Read the model definition and answer for the solid it produces. Units are mm, in the model's axes. A direction names the side the tool comes from. Coordinates: 2 decimals unless noted, no trailing zeros. Loops run counter-clockwise (first coordinate to the right, second up) from the corner with the lowest first, then second, coordinate; pieces in that order, holes last. Notation, with made-up numbers: (7.5, 36) - (44.5, 36) arc R29 cw to (44.5, 58) - close; hole circle Ø1 at (43, 53). An arc over 180 degrees is marked (long way). One line per item, written item: value. Start each with the question number.
from build123d import *

# Parameters (mm, degrees)
SKETCH_1_W               = 35
SKETCH_1_H               = 70
EXTRUDE_1_DEPTH          = 6
SKETCH_1_W_2             = 26
EXTRUDE_1_2_DEPTH        = 6
SKETCH_1_3_W             = 14
SKETCH_1_3_H             = 70
EXTRUDE_2_DEPTH          = 120
EXTRUDE_4_DEPTH          = 70
EXTRUDE_7_DEPTH          = 70
SKETCH_7_R               = 3
CUT_EXTRUDE_4_DEPTH      = 121
SKETCH_8_R               = 5
CUT_EXTRUDE_5_DEPTH      = 115
SKETCH_3_R               = 11.1
SKETCH_3_R_2             = 4.1
SKETCH_3_R_3             = 2
CUT_EXTRUDE_8_DEPTH      = 36
CUT_EXTRUDE_8_DEPTH_BACK = 41
SKETCH_10_W              = 75
SKETCH_10_H              = 24
EXTRUDE_8_DEPTH          = 6
SKETCH_11_R              = 3
CUT_EXTRUDE_9_DEPTH      = 6
SKETCH_12_W              = 56.46589335
SKETCH_12_H              = 70
CUT_EXTRUDE_10_DEPTH     = 60
FILLET_1_R               = 5


with BuildPart() as part:
    # Sketch 1 → Extrude 1 (new body)
    with BuildSketch(Plane(origin=(0, 0, 0), x_dir=(1, 0, 0), z_dir=(0, 1, 0))):
        with Locations((17.5, -35)):
            Rectangle(SKETCH_1_W, SKETCH_1_H)
    extrude(amount=EXTRUDE_1_DEPTH)



with BuildPart() as body_2:
    # Sketch 1 → Extrude 1 2 (new body)
    with BuildSketch(Plane(origin=(0, 0, 0), x_dir=(1, 0, 0), z_dir=(0, 1, 0))):
        with Locations((62, -35)):
            Rectangle(SKETCH_1_W_2, SKETCH_1_H)
    extrude(amount=EXTRUDE_1_2_DEPTH)


with BuildPart() as part_1:
    add(part.part)

    add(body_2.part)  # Extrude 2 merges body 2
    # Sketch 1_3 → Extrude 2 (add)
    with BuildSketch(Plane(origin=(0, 0, 0), x_dir=(1, 0, 0), z_dir=(0, 1, 0))):
        with Locations((42, -35)):
            Rectangle(SKETCH_1_3_W, SKETCH_1_3_H)
    extrude(amount=EXTRUDE_2_DEPTH)

    # Sketch 4 → Extrude 4 (add, through all)
    with BuildSketch(Plane(origin=(0, 0, 0), x_dir=(-1, 0, 0), z_dir=(0, 0, -1))):
        Polygon((-35, 6), (-15, 6), (-35, 38), align=None)
        Polygon((-60, 6), (-40, 38), (-40, 6), align=None)
    extrude(amount=-EXTRUDE_4_DEPTH)

    # Sketch 9 → Extrude 7 (add, through all)
    with BuildSketch(Plane(origin=(0, 0, 0), x_dir=(-1, 0, 0), z_dir=(0, 0, -1))):
        Polygon((-35, 120), (-15, 6), (-35, 0), align=None)
    extrude(amount=-EXTRUDE_7_DEPTH)

    # Sketch 7 → Cut-Extrude 4 (cut, through all)
    with BuildSketch(Plane.XZ):
        with Locations((12.5, 35)):
            Circle(SKETCH_7_R)
        with Locations((12.5, 60)):
            Circle(SKETCH_7_R)
        with Locations((12.5, 10)):
            Circle(SKETCH_7_R)
        with BuildLine():
            ThreePointArc((65.5, 10), (64.621320344, 12.121320344), (62.5, 13))
            Line((62.5, 13), (62.5, 7))
            ThreePointArc((62.5, 7), (64.621320344, 7.878679656), (65.5, 10))
        make_face()
        with BuildLine():
            Line((62.5, 7), (62.5, 13))
            ThreePointArc((62.5, 13), (59.5, 10), (62.5, 7))
        make_face()
        with BuildLine():
            ThreePointArc((65.5, 35), (64.621320344, 37.121320344), (62.5, 38))
            Line((62.5, 38), (62.5, 32))
            ThreePointArc((62.5, 32), (64.621320344, 32.878679656), (65.5, 35))
        make_face()
        with BuildLine():
            Line((62.5, 32), (62.5, 38))
            ThreePointArc((62.5, 38), (59.5, 35), (62.5, 32))
        make_face()
        with BuildLine():
            ThreePointArc((65.5, 60), (64.621320344, 62.121320344), (62.5, 63))
            Line((62.5, 63), (62.5, 57))
            ThreePointArc((62.5, 57), (64.621320344, 57.878679656), (65.5, 60))
        make_face()
        with BuildLine():
            Line((62.5, 57), (62.5, 63))
            ThreePointArc((62.5, 63), (59.5, 60), (62.5, 57))
        make_face()
    extrude(amount=-CUT_EXTRUDE_4_DEPTH, mode=Mode.SUBTRACT)

    # Sketch 8 → Cut-Extrude 5 (cut)
    with BuildSketch(Plane(origin=(0, 6, 0), x_dir=(1, 0, 0), z_dir=(0, 1, 0))):
        with Locations((12.5, -10)):
            Circle(SKETCH_8_R)
        with Locations((62.5, -10)):
            Circle(SKETCH_8_R)
        with Locations((62.5, -35)):
            Circle(SKETCH_8_R)
        with Locations((62.5, -60)):
            Circle(SKETCH_8_R)
        with Locations((12.5, -35)):
            Circle(SKETCH_8_R)
        with Locations((12.5, -60)):
            Circle(SKETCH_8_R)
    extrude(amount=CUT_EXTRUDE_5_DEPTH, mode=Mode.SUBTRACT)

    # Sketch 3 → Cut-Extrude 8 (cut, two sides)
    with BuildSketch(Plane.ZY.offset(-35)) as cut_extrude_8_sk:
        with Locations((35, 86)):
            Circle(SKETCH_3_R)
        with Locations((35, 105.25)):
            Circle(SKETCH_3_R_2)
        with Locations((35, 115)):
            Circle(SKETCH_3_R_3)
        with Locations((60.11473671, 71.5)):
            Circle(SKETCH_3_R_3)
        with Locations((9.88526329, 71.5)):
            Circle(SKETCH_3_R_3)
    extrude(amount=CUT_EXTRUDE_8_DEPTH, mode=Mode.SUBTRACT)
    extrude(cut_extrude_8_sk.sketch, amount=-CUT_EXTRUDE_8_DEPTH_BACK, mode=Mode.SUBTRACT)

    # Sketch 10 → Extrude 8 (add)
    with BuildSketch(Plane.XZ):
        with Locations((37.5, 82)):
            Rectangle(SKETCH_10_W, SKETCH_10_H)
    extrude_8 = extrude(amount=-EXTRUDE_8_DEPTH)

    # Sketch 11 → Cut-Extrude 9 (cut)
    with BuildSketch(Plane(origin=(0, 6, 0), x_dir=(1, 0, 0), z_dir=(0, 1, 0))):
        with Locations((37.5, -85)):
            Circle(SKETCH_11_R)
    cut_extrude_9 = extrude(amount=-CUT_EXTRUDE_9_DEPTH, mode=Mode.SUBTRACT)

    # Mirror 1: Extrude 8, Cut-Extrude 9 across plane
    add(extrude_8.mirror(Plane.XY.offset(35)))
    add(cut_extrude_9.mirror(Plane.XY.offset(35)), mode=Mode.SUBTRACT)

    # Sketch 12 → Cut-Extrude 10 (cut)
    with BuildSketch(Plane(origin=(0, 120, 0), x_dir=(1, 0, 0), z_dir=(0, 1, 0))):
        with Locations((6.767053325, -35)):
            Rectangle(SKETCH_12_W, SKETCH_12_H)
    extrude(amount=-CUT_EXTRUDE_10_DEPTH, mode=Mode.SUBTRACT)

    # Fillet 1
    fillet_1_edges = [part_1.edges().sort_by_distance(p)[0] for p in [
        (24.473684211, 60, 35),
        (35, 60, 35),
    ]]
    fillet(fillet_1_edges, radius=FILLET_1_R)


solid = part_1.part
1) Section C-C, the plane x = 64 is taken. Determine the outline of the cut face in (y, z), and give its area (3 significant figures).
2) Straight lines are drawn through the part: L1, parallel to Y at x = 43.25, z = 35; L2, parallel to Z at x = 12.5, y = 3.8; L3, parallel to X at y = 4.15, z = 85. For each, find the intervals that lie inside material, in ascending order.
3) Determine the mould class of faces 1 (the cylindrical face through (33, 61, 35)), 2 (the cylindrical face through (34.5, 3, -14.9)), 3 (the cylindrical face through (41.902, 73.483, 9.625)) for opening direction Y: released by +Y, released by -Y, zero draft, split by the parting line, or undercut.
4) For faces 4 (the flat face through (37, 51, 0)), 5 (the flat face through (37, 51, 70)), 6 (the cylindrical face through (17.5, 11.4, 10.1)), determine the directions among +Z, -Z, +X, -X, +Y, -Y from which every point of the face is accessible in a straight line to the end or side of a thin tool.
5) Section D-D, the plane x = 47 is taken. Determine the outline of the cut face in (y, z).
6) Flat-ended cylindrical pins translate along their axes: P1, Ø4.5, axis at y = 115, z = 35, coming from the +X side; P2, Ø9.5, axis at x = 12.5, z = 10, coming from the +Y side; P3, Ø0.7, axis at x = 29.5, z = 30, coming from the +Y side. Find the tip coordinate at first contact, or state that the pin passes through.
7) Section B-B, the plane y = 105.25 is taken. Determine the outline of the cut face in (x, z), and give its area (3 significant figures).
8) Section A-A, the plane z = 85 is taken. Determine the outline of the cut face in (x, y).
Answer below:
1. outline: (0, -24) - (6, -24) - (6, 7.4) - (0, 7.4) - close; (0, 12.6) - (6, 12.6) - (6, 32.4) - (0, 32.4) - close; (0, 37.6) - (6, 37.6) - (6, 57.4) - (0, 57.4) - close; (0, 62.6) - (6, 62.6) - (6, 94) - (0, 94) - close
1. area: 614 mm2
2. L1: 0 to 74.9, 97.1 to 101.15, 109.35 to 113, 117 to 120
2. L2: -24 to 7, 13 to 32, 38 to 57, 63 to 94
2. L3: 0 to 34.5, 40.5 to 75
3. face 1: released by +Y
3. face 2: zero draft
3. face 3: undercut
4. face 4: -Z, +X, -X, +Y
4. face 5: +Z, +X, -X, +Y
4. face 6: -X, +Y
5. outline: (0, -24) - (6, -24) - (6, 0) - (120, 0) - (120, 70) - (6, 70) - (6, 94) - (0, 94) - close; hole circle Ø4 at (71.5, 9.89); hole circle Ø4 at (71.5, 60.11); hole circle Ø22.2 at (86, 35); hole circle Ø8.2 at (105.25, 35); hole circle Ø4 at (115, 35)
6. P1: x = 49
6. P2: y = 6
6. P3: y = 60
7. outline: (35, 0) - (49, 0) - (49, 30.9) - (35, 30.9) - close; (35, 39.1) - (49, 39.1) - (49, 70) - (35, 70) - close
7. area: 865 mm2
8. outline: (0, 0) - (34.5, 0) - (34.5, 6) - (0, 6) - close; (40.5, 0) - (75, 0) - (75, 6) - (40.5, 6) - close
